Input: dimensioned drawing with shaded views. Units: mm. Origin: part minimum x, y, z. Coordinates: 2 decimals unless noted, no trailing zeros. Loops run counter-clockwise (first coordinate to the right, second up) from the corner with the lowest first, then second, coordinate; pieces in that order, holes last.
Item 1: Section query B-B, the plane z = 65. Return the cut outline in (x, y).
Item 2: Pin query (flat end, axial travel): pin 1 Ø1 at (x, z) = (60, 42) entering from -Y; pin 2 Ø1.5 at (y, z) = (8, 43) entering from +X; pin 3 Ø1 at (x, z) = (53, 31.5) entering from +Y; pin 4 Ø1.5 at (x, y) = (45.5, 2) entering from -Z. Return the tip coordinate at first contact, or that it passes through.
Item 3: Section query C-C, the plane x = 18.5. Return the cut outline in (y, z), then the cut area to 3 significant figures.
Item 4: Line query: probe 1 along X at (y, z) = (8.45, 36); probe 2 along Z at (x, y) = (36, 4.15); probe 3 along X at (y, z) = (4.4, 65). Output: solid intervals per line, ascending.
Item 5: Section query A-A, the plane x = 36. Return the cut outline in (y, z).
Item 6: Section query D-D, the plane z = 36. Return the cut outline in (x, y), then the cut area to 3 significant figures.
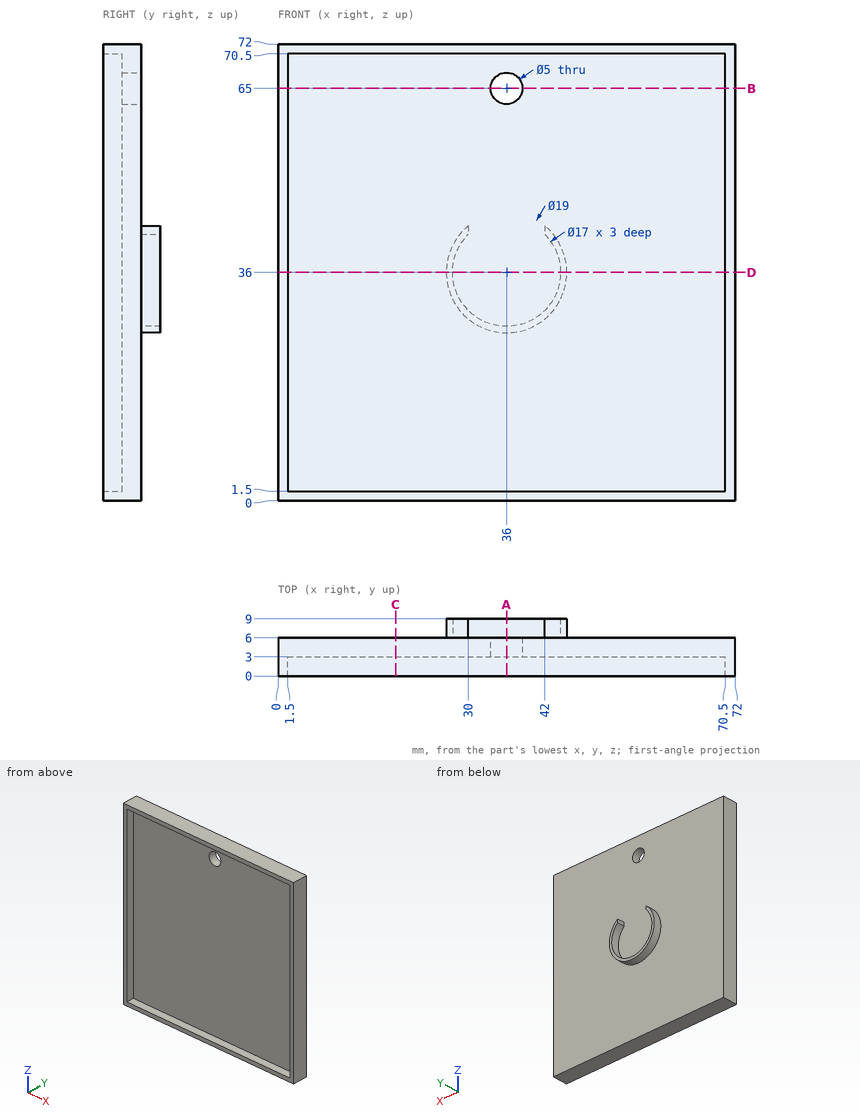
Verdict:
1. outline: (0, 0) - (1.5, 0) - (1.5, 3) - (33.5, 3) - (33.5, 6) - (0, 6) - close; (38.5, 3) - (70.5, 3) - (70.5, 0) - (72, 0) - (72, 6) - (38.5, 6) - close
2. pin 1: stops at y = 3
2. pin 2: stops at x = 43.15
2. pin 3: stops at y = 6
2. pin 4: stops at z = 0
3. outline: (0, 0) - (6, 0) - (6, 72) - (0, 72) - (0, 70.5) - (3, 70.5) - (3, 1.5) - (0, 1.5) - close
3. area: 225 mm2
4. probe 1: x = 26.5 to 27.5, 44.5 to 45.5
4. probe 2: z = 0 to 62.5, 67.5 to 72
4. probe 3: x = 0 to 33.5, 38.5 to 72
5. outline: (0, 0) - (6, 0) - (6, 26.5) - (9, 26.5) - (9, 27.5) - (6, 27.5) - (6, 62.5) - (3, 62.5) - (3, 1.5) - (0, 1.5) - close; (0, 70.5) - (3, 70.5) - (3, 67.5) - (6, 67.5) - (6, 72) - (0, 72) - close
6. outline: (0, 0) - (1.5, 0) - (1.5, 3) - (70.5, 3) - (70.5, 0) - (72, 0) - (72, 6) - (45.5, 6) - (45.5, 9) - (44.5, 9) - (44.5, 6) - (27.5, 6) - (27.5, 9) - (26.5, 9) - (26.5, 6) - (0, 6) - close
6. area: 231 mm2
